For this review, take the finished solid that the model builds, in its own axes (mm). Coordinates: 2 decimals unless noted, no trailing zeros.
```python
from build123d import *

# Parameters (mm, degrees)
SKETCH1_R               = 73.7362
MAIN_DEPTH              = 25.4
SKETCH2_R               = 82.55
SHOULDER_DEPTH          = 9.525
F_1_4_CLEARANCE_HOLE1_D = 6.7564
F_1_2_CLEARANCE_HOLE1_D = 13.09624
CHAMFER1_SIZE           = 0.762


with BuildPart() as part:
    # Sketch1 → Main (new body)
    with BuildSketch(Plane.XY):
        Circle(SKETCH1_R)
    extrude(amount=MAIN_DEPTH)

    # Sketch2 → Shoulder (add)
    with BuildSketch(Plane.XY.offset(25.4)):
        with Locations(Location((0, 0, 0), (0, 0, 180))):
            Circle(SKETCH2_R)
    extrude(amount=SHOULDER_DEPTH)

    # 1/4 Clearance Hole1 (through all)
    with Locations(Plane.XY.offset(34.925)):
        with Locations((26.940768363, 26.940768363), (0, 38.1), (38.1, 0), (0, -38.1), (-38.1, 0), (26.940768363, -26.940768363), (-26.940768363, -26.940768363), (-26.940768363, 26.940768363), (-19.05, 32.995567884), (19.05, 32.995567884), (32.995567884, 19.05), (-32.995567884, 19.05), (-32.995567884, -19.05), (-19.05, -32.995567884), (19.05, -32.995567884), (32.995567884, -19.05)):
            Hole(F_1_4_CLEARANCE_HOLE1_D / 2)

    # 1/2 Clearance Hole1 (through all)
    with Locations(Plane.XY.offset(34.925)):
        with Locations((0, 0), (124.453596133, 85.444632909)):
            Hole(F_1_2_CLEARANCE_HOLE1_D / 2)

    # Chamfer1
    chamfer1_edges = [part.edges().sort_by_distance(p)[0] for p in [
        (30.318968363, -26.940768363, 0),
        (-34.7218, 0, 34.925),
        (-34.7218, 0, 0),
        (3.3782, -38.1, 34.925),
        (3.3782, -38.1, 0),
        (41.4782, 0, 34.925),
        (41.4782, 0, 0),
        (3.3782, 38.1, 34.925),
        (3.3782, 38.1, 0),
        (6.54812, 0, 34.925),
        (6.54812, 0, 0),
        (-73.7362, 0, 0),
        (30.318968363, 26.940768363, 34.925),
        (30.318968363, 26.940768363, 0),
        (36.373767884, -19.05, 34.925),
        (36.373767884, -19.05, 0),
        (22.4282, -32.995567884, 34.925),
        (22.4282, -32.995567884, 0),
        (-15.6718, -32.995567884, 34.925),
        (-15.6718, -32.995567884, 0),
        (-29.617367884, -19.05, 34.925),
        (-29.617367884, -19.05, 0),
        (-29.617367884, 19.05, 34.925),
        (-29.617367884, 19.05, 0),
        (82.55, 0, 25.4),
        (82.55, 0, 34.925),
        (36.373767884, 19.05, 34.925),
        (36.373767884, 19.05, 0),
        (22.4282, 32.995567884, 34.925),
        (22.4282, 32.995567884, 0),
        (-15.6718, 32.995567884, 34.925),
        (-15.6718, 32.995567884, 0),
        (-23.562568363, 26.940768363, 34.925),
        (-23.562568363, 26.940768363, 0),
        (-23.562568363, -26.940768363, 34.925),
        (-23.562568363, -26.940768363, 0),
        (30.318968363, -26.940768363, 34.925),
    ]]
    chamfer(chamfer1_edges, length=CHAMFER1_SIZE)


solid = part.part
```
Q1. Draft analysis for pull direction X (two halves, no side actions). For faces 1 (the cylindrical face through (10.746, -81.848, 30.106)), 2 (the cylindrical face through (29.875, 17.756, 17.229)), 3 (the flat face through (12, -73, 25.4)), state which applies: +X half, -X half, draft (parallel to the pull), parting line (faces both ways), or undercut.
Ans:
face 1: parting line
face 2: undercut
face 3: draft
Q2. For probe 1 along X at (y, z) = (32.5, 6); probe 2 along X at (y, z) = (-19, 21); probe 3 along Y at (x, z) = (21.5, 8), list the stretches that pass through material, from the lowest coordinate up.
Ans:
probe 1: x = -66.19 to -22.39, -15.71 to 15.71, 22.39 to 66.19
probe 2: x = -71.25 to -36.37, -29.62 to 29.62, 36.37 to 71.25
probe 3: y = -70.53 to -35.32, -30.67 to 30.67, 35.32 to 70.53
Q3. Clearance check with flat-ended pins moving along their axes: pin 1 Ø10 at (y, z) = (7, 6.5) entering from -X; pin 2 Ø1.5 at (x, z) = (12.5, 29.5) entering from -Y; pin 3 Ø1 at (y, z) = (39, 18) entering from +X. State where each tip first meets the part, or that it passes through.
Ans:
pin 1: stops at x = -73.71
pin 2: stops at y = -81.71
pin 3: stops at x = 62.89
Q4. Add section A-A (x = 0). Give the number of separate pieces and of enclosed holes in the cut face, then the cut area to 3 significant figures.
Ans:
separate pieces: 4
enclosed holes: 0
area: 4,380 mm2
